The figure shows three views and two pictorial views of one solid part (mm, origin at its lowest corner). Answer the questions. Coordinates: 2 decimals unless noted, no trailing zeros.
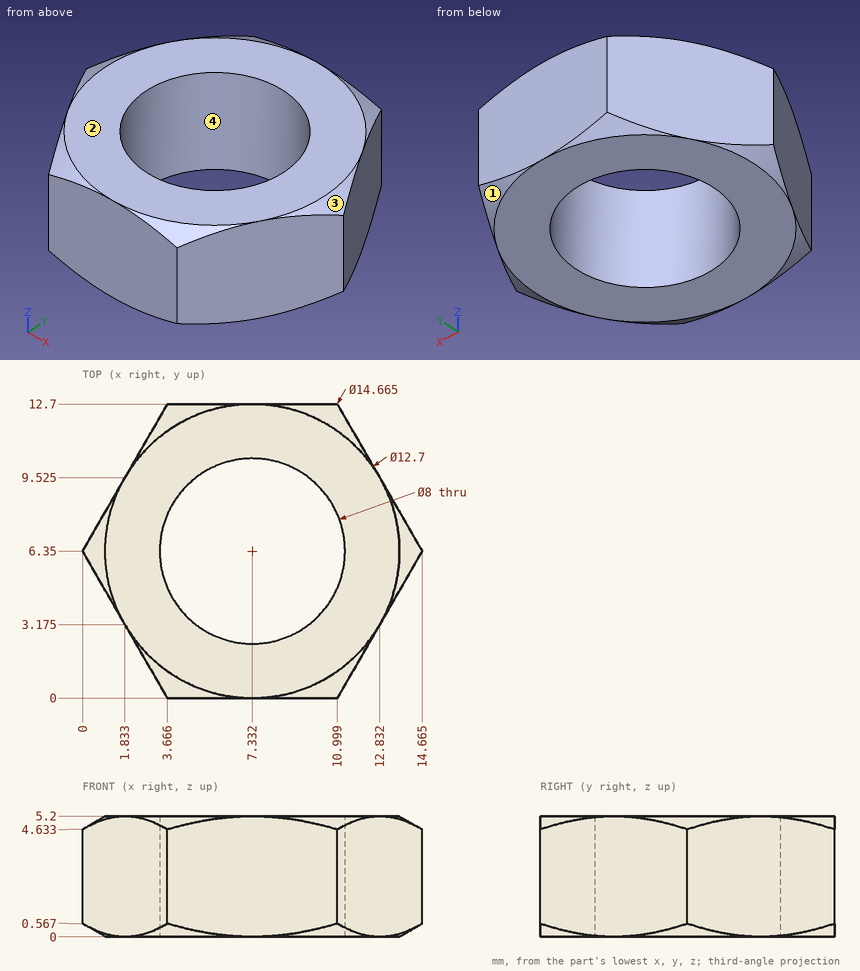
1) The mould has two halves that part along Y. Classify the marked faces 1, 2, 3 and 4: released by +Y, released by -Y, zero draft, split by the parting line, or undercut.
2) Straight lines are drawn through the part: probe 1 along X at (y, z) = (5, 3.35) (1 decimal); probe 2 along Y at (x, z) = (10.5, 0.6) (1 decimal); probe 3 along Y at (x, z) = (5, 2.15). For each, find the intervals that lie inside material, in ascending order.
3) Each of these flat-tipped pins is pushed along its axis until it touches: P1, Ø1.5, axis at y = 3, z = 3, coming from the +X side; P2, Ø1, axis at y = 5, z = 2, coming from the -X side. Where does it stop, or does it pass through?
Working result:
1. face 1: released by +Y
1. face 2: zero draft
1. face 3: split by the parting line
1. face 4: undercut
2. probe 1: x = 0.8 to 3.6, 11.1 to 13.9
2. probe 2: y = 0 to 3.9, 8.8 to 12.7
2. probe 3: y = 0 to 3.1, 9.6 to 12.7
3. P1: stops at x = 13.16
3. P2: stops at x = 0.49
